Geometry: final body of the model. Coordinates: model frame, mm. Face numbers are marked on the shaded views. A direction names the side the tool comes from. Give positions to 0.01 mm unless a question says otherwise; leave off trailing zeros. Order: outer loops, then holes, each group sorted by start corner. A loop starts at its lowest first (then second) coordinate and runs counter-clockwise, first axis right, second up. Notation, with made-up numbers: (38.5, -27) - (61.5, -27) arc R32 ccw to (61.5, 7) - close; hole circle Ø1 at (35.25, 53.25). An arc over 180 degrees is marked (long way). Write item = value, one per line. Start each with the question number.
from build123d import *

# Parameters (mm, degrees)
BOSS_EXTRUDE1_DEPTH     = 40
FILLET1_R               = 10
SKETCH2_R               = 3
CUT_EXTRUDE1_DEPTH      = 30
CUT_EXTRUDE2_DEPTH      = 56.598274214
CUT_EXTRUDE2_DEPTH_BACK = 56.598274214
SKETCH4_R               = 10.65
SKETCH3_R               = 3
CUT_EXTRUDE3_DEPTH      = 15
SKETCH10_W              = 8
SKETCH10_H              = 8
CUT_EXTRUDE4_DEPTH      = 22
CUT_EXTRUDE5_DEPTH      = 1
CUT_EXTRUDE6_DEPTH      = 1


with BuildPart() as part:
    # Sketch1 → Boss-Extrude1 (new body)
    with BuildSketch(Plane(origin=(0, 0, 0), x_dir=(1, 0, 0), z_dir=(0, 1, 0))):
        with BuildLine():
            Line((0, 22.5), (30, 22.5))
            Line((30, 22.5), (30, -22.5))
            Line((30, -22.5), (0, -22.5))
            ThreePointArc((0, -22.5), (-13.205112646, -18.217436702), (-21.38340478, -7))
            Line((-21.38340478, -7), (-31.38340478, -7))
            Line((-31.38340478, -7), (-31.38340478, -1))
            Line((-31.38340478, -1), (-14.966629547, -1))
            ThreePointArc((-14.966629547, -1), (15, 0), (-14.966629547, 1))
            Line((-14.966629547, 1), (-31.38340478, 1))
            Line((-31.38340478, 1), (-31.38340478, 7))
            Line((-31.38340478, 7), (-21.38340478, 7))
            ThreePointArc((-21.38340478, 7), (-13.205112646, 18.217436702), (0, 22.5))
        make_face()
    extrude(amount=BOSS_EXTRUDE1_DEPTH)

    # Fillet1
    fillet1_edges = [part.edges().sort_by_distance(p)[0] for p in [
        (-31.38340478, 40, -4),
        (-31.38340478, 0, -4),
        (-31.38340478, 0, 4),
        (-31.38340478, 40, 4),
    ]]
    fillet(fillet1_edges, radius=FILLET1_R)

    # Sketch2 → Cut-Extrude1 (cut)
    with BuildSketch(Plane.XY.offset(7)):
        with Locations((-25.88340478, 32.5)):
            Circle(SKETCH2_R)
        with Locations((-25.88340478, 7.5)):
            Circle(SKETCH2_R)
    extrude(amount=-CUT_EXTRUDE1_DEPTH, mode=Mode.SUBTRACT)

    # Sketch4 → Cut-Extrude2 (cut, two sides: drawn at the far end of the back side and taken through both)
    with BuildSketch(Plane.XY.offset(-CUT_EXTRUDE2_DEPTH_BACK)):
        with Locations((30, 20)):
            Circle(SKETCH4_R)
    extrude(amount=CUT_EXTRUDE2_DEPTH + CUT_EXTRUDE2_DEPTH_BACK, mode=Mode.SUBTRACT)

    # Sketch3 → Cut-Extrude3 (cut)
    with BuildSketch(Plane(origin=(30, 0, 0), x_dir=(0, 0, -1), z_dir=(1, 0, 0))):
        with Locations((-17.8, 35.3)):
            Circle(SKETCH3_R)
        with Locations((17.8, 35.3)):
            Circle(SKETCH3_R)
        with Locations((17.8, 4.7)):
            Circle(SKETCH3_R)
        with Locations((-17.8, 4.7)):
            Circle(SKETCH3_R)
    extrude(amount=-CUT_EXTRUDE3_DEPTH, mode=Mode.SUBTRACT)

    # Sketch10 → Cut-Extrude4 (cut)
    with BuildSketch(Plane.ZY.offset(31.38340478)):
        with Locations((-16, 29)):
            Rectangle(SKETCH10_W, SKETCH10_H)
        with Locations((16, 29)):
            Rectangle(SKETCH10_W, SKETCH10_H)
        with Locations((16, 11)):
            Rectangle(SKETCH10_W, SKETCH10_H)
        with Locations((-16, 11)):
            Rectangle(SKETCH10_W, SKETCH10_H)
    extrude(amount=-CUT_EXTRUDE4_DEPTH, mode=Mode.SUBTRACT)

    # Sketch11 → Cut-Extrude5 (cut)
    with BuildSketch(Plane(origin=(0, 40, 0), x_dir=(1, 0, 0), z_dir=(0, 1, 0))):
        with BuildLine():
            Line((25, 20), (25, -20))
            Line((25, -20), (0, -20))
            Line((0, -20), (0, -17.5))
            ThreePointArc((0, -17.5), (17.5, 0), (0, 17.5))
            Line((0, 17.5), (0, 20))
            Line((0, 20), (25, 20))
        make_face()
    cut_extrude5 = extrude(amount=-CUT_EXTRUDE5_DEPTH, mode=Mode.SUBTRACT)

    # Sketch14 → Cut-Extrude6 (cut)
    with BuildSketch(Plane.XY.offset(22.5)):
        with BuildLine():
            Line((7.05e-07, 24.999999636), (2.260270537, 24.999999636))
            ThreePointArc((2.260270537, 24.999999636), (7.080945531, 26.238658837), (10.707385838, 29.647781115))
            ThreePointArc((10.707385838, 29.647781115), (17.545274901, 35.950998172), (26.616595925, 37.999999636))
            Line((26.616595925, 37.999999636), (26.616595925, 31.999999636))
            ThreePointArc((26.616595925, 31.999999636), (17.616595925, 19.999999636), (26.616595925, 7.999999636))
            Line((26.616595925, 7.999999636), (26.616595925, 1.999999636))
            ThreePointArc((26.616595925, 1.999999636), (17.545274901, 4.0490011), (10.707385838, 10.352218158))
            ThreePointArc((10.707385838, 10.352218158), (7.080945531, 13.761340436), (2.260270537, 14.999999636))
            Line((2.260270537, 14.999999636), (7.05e-07, 14.999999636))
            Line((7.05e-07, 14.999999636), (7.05e-07, 24.999999636))
        make_face()
    cut_extrude6 = extrude(amount=-CUT_EXTRUDE6_DEPTH, mode=Mode.SUBTRACT)

    # Mirror3: Cut-Extrude6 across plane
    add(cut_extrude6.mirror(Plane.XY), mode=Mode.SUBTRACT)

    # Mirror4: Cut-Extrude5 across plane
    add(cut_extrude5.mirror(Plane.ZX.offset(20)), mode=Mode.SUBTRACT)


solid = part.part
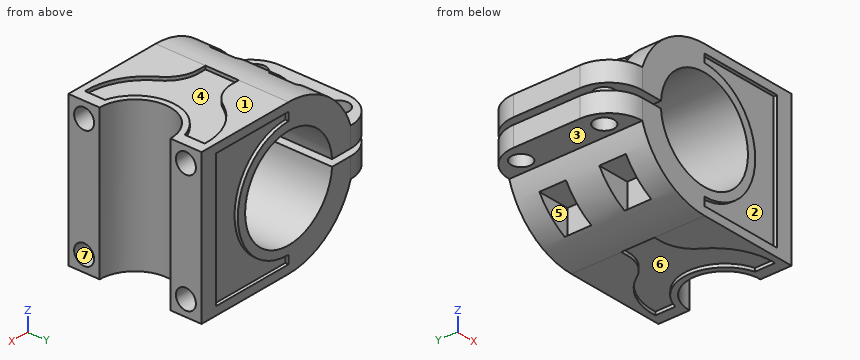
Q1. Section B-B, the plane y = 20. Return the cut outline in (x, z), then the cut area to 3 significant figures.
Q2. Section D-D, the plane x = 23. Count the separate pieces of the cut face and the enclosed holes in it, then the cut area to 3 significant figures.
Q3. Contact query for flat-ended pins moving along their axis: pin 1 (5 mm diameter, centred on x = -25, y = 6, fed in from -Z); pin 2 (3 mm diameter, centred on x = -22, y = 29.5, fed in from -Z); pin 3 (5 mm diameter, centred on x = 21, z = -1, fed in from +Y). Output: stop coordinate, or through.
Q4. Pull-direction query (Z, two-part tool) for the marked faces 1, 2 and 3; classes: +Z half, -Z half, draft (parallel to the pull), parting line (faces both ways), or undercut.
Q5. Section C-C, the plane z = 0. Return the cut outline in (x, y), then the cut area to 3 significant figures.
Q6. Material intervals for line 1 along Y through (x, z) = (18.75, 17.8); line 2 along Y through (x, z) = (-14, -14); line 3 along Z through (x, y) = (-22.5, 3), sorted ascending. Write a range as from..to.
Q7. Set-up query: the marked faces 4, 5, 6 and 7. Return all of +Z, -Z, +X, -X, +Y, -Y with unobstructed straight access to the full face (end or side cutting, diameter ignored); none if empty.
The answers:
q1.outline = (-31.38, -7) - (-21.38, -7) arc R22.5 ccw to (0, -22.5) - (0, -21.5) - (17.62, -21.5) - (17.62, -22.5) - (19.35, -22.5) - (19.35, 22.5) - (17.62, 22.5) - (17.62, 21.5) - (0, 21.5) - (0, 22.5) arc R22.5 ccw to (-21.38, 7) - (-31.38, 7) - (-31.38, 1) - (-14.97, 1) arc R15 cw (long way) to (-14.97, -1) - (-31.38, -1) - close
q1.area = 1,020 mm²
q2.separate_pieces = 2
q2.enclosed_holes = 4
q2.area = 855 mm²
q3.pin_1 = -7
q3.pin_2 = -9.27
q3.pin_3 = 39
q4.face_1 = +Z half
q4.face_2 = undercut
q4.face_3 = -Z half
q5.outline = (15, 0) - (17.5, 0) - (17.5, 1) - (25, 1) - (25, 0) - (30, 0) - (30, 9.35) arc R10.65 cw to (30, 30.65) - (30, 40) - (25, 40) - (25, 39) - (17.5, 39) - (17.5, 40) - (15, 40) - close
q5.area = 407 mm²
q6.line_1 = 1..1.7, 7.7..32.3, 38.3..39
q6.line_2 = 0..7, 15..25, 33..40
q6.line_3 = -7..-1, 1..7
q7.face_4 = +Z
q7.face_5 = -X
q7.face_6 = -Z
q7.face_7 = +X
